Model file for the job. Use its own axes, mm. A direction names the side the tool comes from. Round coordinates to 2 decimals unless told otherwise and drop trailing zeros. Write each loop counter-clockwise with the first axis right and the second up, starting at its lowest first coordinate (ties: lowest second). Pieces come first, ordered by that corner, then holes. Notation, with made-up numbers: (-1, 38.5) - (42, 38.5) arc R20 cw to (42, 51.5) - close; hole circle Ø8 at (59.5, 39.5). An arc over 180 degrees is marked (long way). Answer as a JSON object with one key per item and string values. Group by question number.
Autodesk Inventor part; units mm, degrees
ref_plane "YZ Plane" through (0, 0, 0) normal (1, 0, 0) x (0, 1, 0)
ref_plane "XZ Plane" through (0, 0, 0) normal (0, 1, 0) x (-1, 0, 0)
ref_plane "XY Plane" through (0, 0, 0) normal (0, 0, 1) x (1, 0, 0)
sketch "Sketch1" plane through (0, 0, 0) normal (0, 0, 1) x (1, 0, 0)
  line L0 (-27.5, -4.5) -> (27.5, -4.5)
  line L1 (27.5, -4.5) -> (27.5, 4.5)
  line L2 (27.5, 4.5) -> (-27.5, 4.5)
  line L3 (-27.5, 4.5) -> (-27.5, -4.5)
  line L4 (-27.5, -4.5) -> (27.5, 4.5) construction
  line L5 (27.5, -4.5) -> (-27.5, 4.5) construction
  point P0 (0, 0)
  dimension "d0" = 55
  dimension "d1" = 9
extrude "Extrusion1" add sketch "Sketch1" along normal mid plane 4
sketch "Sketch2" plane through (0, 0, 2) normal (0, 0, 1) x (1, 0, 0)
  line L0 (-27.5, 4.5) -> (-27.5, -4.5)
  line L1 (-27.5, -3.25) -> (-4.5, -3.25)
  line L2 (-4.5, -3.25) -> (-4.5, 3.25)
  line L3 (-4.5, 3.25) -> (-27.5, 3.25)
  line L4 (-27.5, 3.25) -> (-27.5, -3.25)
  point P0 (0, 0)
  point P1 (-4.5, 0)
  dimension "d4" = 23
  dimension "d5" = 6.5
extrude "Extrusion2" cut sketch "Sketch2" against normal blind 2
sketch "Sketch3" plane through (0, 0, 0) normal (0, 0, 1) x (1, 0, 0)
  circle A0 centre (-21.5, 0) radius 2.5
  line L0 (-27.5, -3.25) -> (-27.5, 3.25)
  point P0 (0, 0)
  dimension "d8" = 5
  dimension "d13" = 6
extrude "Extrusion3" cut sketch "Sketch3" against normal blind 2
fillet "Fillet1" radius 4 2 edges at (27.5, 4.5, 0) (27.5, -4.5, 0)
fillet "Fillet2" radius 4 2 edges at (-27.5, 4.5, 0) (-27.5, -4.5, 0)
properties part number "Servo Arm"
(1) Slice it at A-A (x = -21.5). Write the cut outline in (y, z), then the cut area to 3 significant figures.
(2) Slice it at C-C (y = 0). Write the cut outline in (x, z).
(3) Slice it at B-B (z = -1.25). Write the cut outline in (x, y).
(4) Drill centre lines: line 1 (Y direction, x = -21.5, z = -1.15); line 2 (X direction, y = 0.75, z = 1.6); line 3 (Z direction, x = -10, y = -2.75). Where is each one in solid material? Low to high. Write a range as from..to.
(5) Flat gauge pin, fed straight in: pin 1 (2 mm diameter, centred on y = 0, z = 0.5, fed in from -X). Where does the tip first touch, or does it go through?
(6) Slice it at D-D (z = 1). Write the cut outline in (x, y), then the cut area to 3 significant figures.
(7) Pull direction Y, two halves, no side cores. Call faces 3 (the flat face through (-16, -3.25, 1)), 4 (the cylindrical face through (-25.83, 3.75, -0.47)), 5 (the cylindrical face through (-25.83, -3.75, -0.42)): pulls with the +Y half, pulls with the -Y half, needs draft (parallel to the pull), parting line crosses it, or undercut.
(8) 3-axis set-ups, long thin cutter, end or side, ignore diameter. For faces 1 (the flat face through (0, -4.5, 0)), 2 (the flat face through (-16, 0, 0)): which of +Z, -Z, +X, -X, +Y, -Y reach the whole face in a straight line?
Answer:
{
 "1": {"outline": "(-4.5, -2) - (-2.5, -2) - (-2.5, 0) - (-3.25, 0) - (-3.25, 2) - (-4.5, 2) - close; (2.5, -2) - (4.5, -2) - (4.5, 2) - (3.25, 2) - (3.25, 0) - (2.5, 0) - close", "area": "13.0 mm²"},
 "2": {"outline": "(-27.5, -2) - (-24, -2) - (-24, 0) - (-27.5, 0) - close; (-19, -2) - (27.5, -2) - (27.5, 2) - (-4.5, 2) - (-4.5, 0) - (-19, 0) - close"},
 "3": {"outline": "(-27.5, -0.5) arc R4 ccw to (-23.5, -4.5) - (23.5, -4.5) arc R4 ccw to (27.5, -0.5) - (27.5, 0.5) arc R4 ccw to (23.5, 4.5) - (-23.5, 4.5) arc R4 ccw to (-27.5, 0.5) - close; hole circle Ø5 at (-21.5, 0)"},
 "4": {"line 1": "-4.5..-2.5, 2.5..4.5", "line 2": "-4.5..27.49", "line 3": "-2..0"},
 "5": {"pin 1": "x = -27.5"},
 "6": {"outline": "(-26.4, -3.25) arc R4 ccw to (-23.5, -4.5) - (23.5, -4.5) arc R4 ccw to (27.5, -0.5) - (27.5, 0.5) arc R4 ccw to (23.5, 4.5) - (-23.5, 4.5) arc R4 ccw to (-26.4, 3.25) - (-4.5, 3.25) - (-4.5, -3.25) - close", "area": "334 mm²"},
 "7": {"face 3": "undercut", "face 4": "pulls with the +Y half", "face 5": "pulls with the -Y half"},
 "8": {"face 1": "+Z, -Z, +X, -X, -Y", "face 2": "+Z, -X"}
}
